Can you work these out from the model? Positions are in its coordinate system, mm. Give positions to 0.01 mm unless a question says otherwise; leave off trailing zeros. Write each loop counter-clockwise with the first axis right and the second up, starting at its lowest first coordinate (ties: lowest second). Pieces come first, ordered by that corner, then holes. Notation, with made-up numbers: (-28.75, 48) -> (-6.75, 48) arc R11 ccw to (-6.75, 52) -> close; hole circle Ø5 at (49, -10.75). An arc over 180 degrees is marked (long way). One line per item, written item: value.
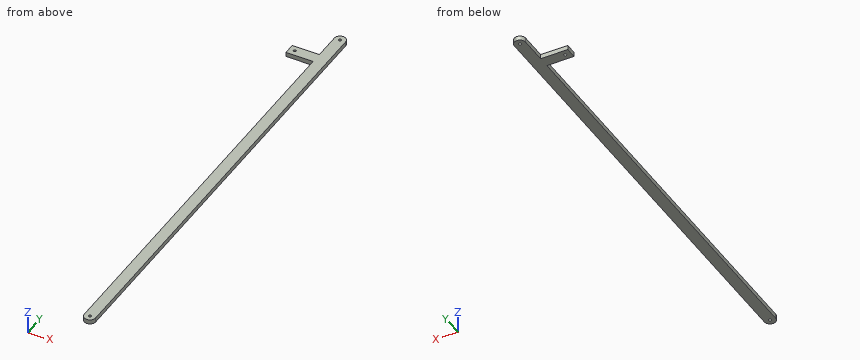
from build123d import *

# Parameters (mm, degrees)
SKETCH1_R           = 3
BOSS_EXTRUDE1_DEPTH = 10


with BuildPart() as part:
    # Sketch1 → Boss-Extrude1 (new body)
    with BuildSketch(Plane.XY):
        with BuildLine():
            Line((-12.5, 0), (-12.5, -60))
            Line((-12.5, -60), (-72.5, -60))
            Line((-72.5, -60), (-72.5, -85))
            Line((-72.5, -85), (-12.5, -85))
            Line((-12.5, -85), (-12.5, -1000))
            ThreePointArc((-12.5, -1000), (0, -1012.5), (12.5, -1000))
            Line((12.5, -1000), (12.5, 0))
            ThreePointArc((12.5, 0), (0, 12.5), (-12.5, 0))
        make_face()
        Circle(SKETCH1_R, mode=Mode.SUBTRACT)
        with Locations(Location((0, -1000, 0), (0, 0, 180))):
            Circle(SKETCH1_R, mode=Mode.SUBTRACT)
        with Locations((-60, -72.5)):
            Circle(SKETCH1_R, mode=Mode.SUBTRACT)
    extrude(amount=BOSS_EXTRUDE1_DEPTH)


solid = part.part
1) Will these pins go through, and if not, where does the flat tip stop? pin 1 (5 mm diameter, centred on x = -38, z = 6, fed in from -Y); pin 2 (5 mm diameter, centred on x = -56, z = 3, fed in from +Y); pin 3 (6 mm diameter, centred on x = -14, z = 5.5, fed in from -Y); pin 4 (3.5 mm diameter, centred on x = -60, y = -72.5, fed in from -Z).
Answer list:
pin 1: stops at y = -85
pin 2: stops at y = -60
pin 3: stops at y = -1005.94
pin 4: passes through
2) If we section it at B-B (x = -40): Write out the boundary of the cut face in (y, z).
Answer list:
outline: (-85, 0) -> (-60, 0) -> (-60, 10) -> (-85, 10) -> close
3) If we section it at C-C (y = -231): Write out the boundary of the cut face in (x, z).
Answer list:
outline: (-12.5, 0) -> (12.5, 0) -> (12.5, 10) -> (-12.5, 10) -> close
4) If we section it at A-A (z = 7.75): Write out the boundary of the cut face in (x, y).
Answer list:
outline: (-72.5, -85) -> (-12.5, -85) -> (-12.5, -1000) arc R12.5 ccw to (12.5, -1000) -> (12.5, 0) arc R12.5 ccw to (-12.5, 0) -> (-12.5, -60) -> (-72.5, -60) -> close; hole circle Ø6 at (-60, -72.5); hole circle Ø6 at (0, -1000); hole circle Ø6 at (0, 0)
5) I need wall thicknesses on L1, parallel to Y at x = -59, z = 5; L2, parallel to Y at x = -60, z = 4; L3, parallel to X at y = -110.5, z = 3.5. Which ranges of each line are inside material? Lowest first, please.
Answer list:
L1: y = -85 to -75.33, -69.67 to -60
L2: y = -85 to -75.5, -69.5 to -60
L3: x = -12.5 to 12.5
